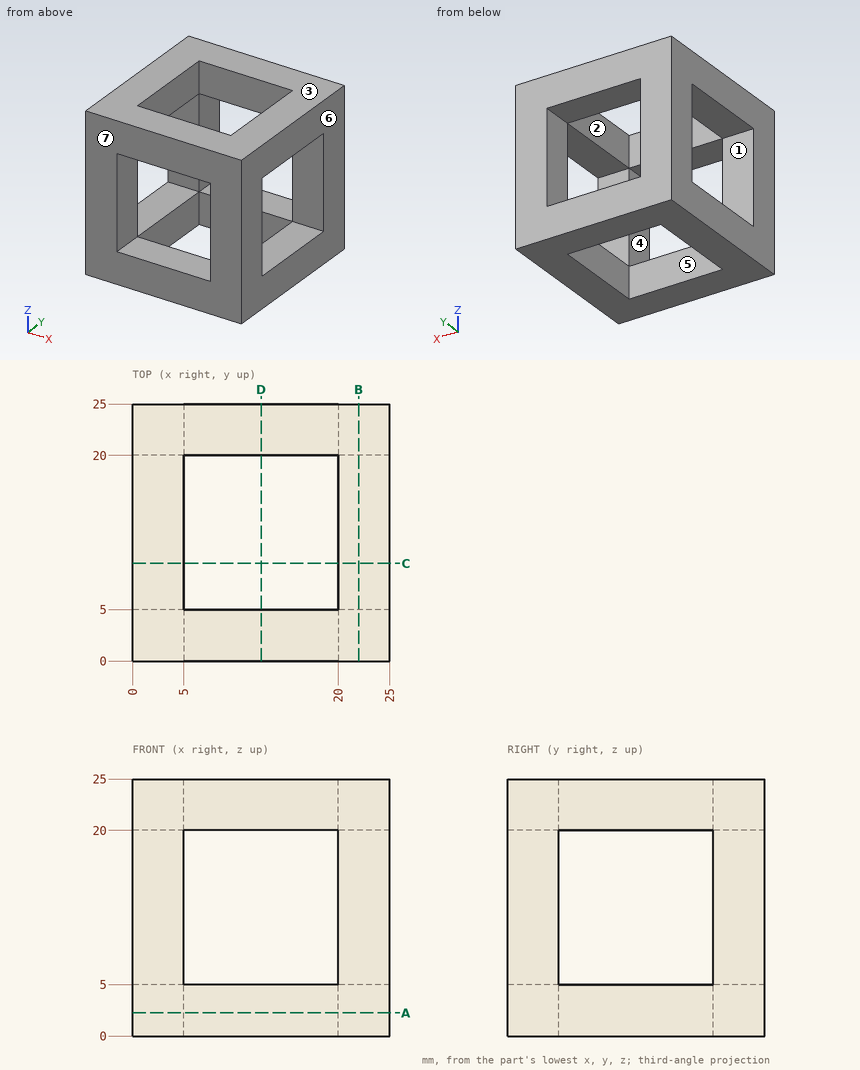
Here's the drawing with two shaded views (mm, measured from the low corner). I have some questions. A direction names the side the tool comes from. Coordinates: 2 decimals unless noted, no trailing zeros. Write each loop counter-clockwise with the first axis right and the second up, starting at its lowest first coordinate (ties: lowest second). Pieces come first, ordered by that corner, then holes. Notation, with made-up numbers: M 87.25,42 L 140.25,42 A21 ccw 140.25,74 Z; hole C -31,-33.75 d8. An arc over 180 degrees is marked long. Answer as CSV lines item,"result".
Item 1: Please list where this line runs through material, in increasing order: line 1 along Y through (x, z) = (12.5, 21.25).
Geometry results:
line 1,"y = 0 to 5, 20 to 25"
Item 2: We'd pull the mould along X, two halves only. Please class the marked faces 5, 6 and 7: +X half, -X half, draft (parallel to the pull), parting line (faces both ways), or undercut.
Geometry results:
face 5,"undercut"
face 6,"+X half"
face 7,"draft"
Item 3: On a 3-axis mill with a long thin cutter (end or side, diameter ignored), from which of +Z, -Z, +X, -X, +Y, -Y can I reach the whole of each face in a straight line? I mean the marked faces 1, 2, 3 and 4. Say none if no direction works.
Geometry results:
face 1,"+X, -X"
face 2,"+Z, -Z"
face 3,"+Z, +X, -X, +Y, -Y"
face 4,"+Y, -Y"
Item 4: Imagine slicing it at A-A on z = 2.25. List the corners of the cut face in (x, y) for me, plus the area to 3 significant figures.
Geometry results:
outline,"M 0,0 L 25,0 L 25,25 L 0,25 Z; hole M 5,5 L 20,5 L 20,20 L 5,20 Z"
area,"400 mm2"
Item 5: Imagine slicing it at C-C on y = 9.5. List the corners of the cut face in (x, z) for me.
Geometry results:
outline,"M 0,0 L 5,0 L 5,5 L 0,5 Z; M 0,20 L 5,20 L 5,25 L 0,25 Z; M 20,0 L 25,0 L 25,5 L 20,5 Z; M 20,20 L 25,20 L 25,25 L 20,25 Z"
Item 6: I'm going to push a flat-ended pin straight in: P1, Ø5.5, axis at x = 14.5, y = 3.5, coming from the -Z side. Where does the tip first touch, or does it pass through?
Geometry results:
P1,"stops at z = 0"
